```python
from build123d import *

# Parameters (mm, degrees)
F0_R     = 11
F1_DEPTH = 15


with BuildPart() as f1:
    # F0 (on Front) → F1 (new body)
    with BuildSketch(Plane.XZ):
        with BuildLine():
            Line((625, -53.625), (625, 53.625))
            Line((625, 53.625), (553.618176, 53.625))
            ThreePointArc((553.618176, 53.625), (525, 27.625), (496.381824, 53.625))
            Line((496.381824, 53.625), (478.618176, 53.625))
            ThreePointArc((478.618176, 53.625), (450, 27.625), (421.381824, 53.625))
            Line((421.381824, 53.625), (403.618176, 53.625))
            ThreePointArc((403.618176, 53.625), (375, 27.625), (346.381824, 53.625))
            Line((346.381824, 53.625), (328.618176, 53.625))
            ThreePointArc((328.618176, 53.625), (300, 27.625), (271.381824, 53.625))
            Line((271.381824, 53.625), (253.618176, 53.625))
            ThreePointArc((253.618176, 53.625), (225, 27.625), (196.381824, 53.625))
            Line((196.381824, 53.625), (178.618176, 53.625))
            ThreePointArc((178.618176, 53.625), (150, 27.625), (121.381824, 53.625))
            Line((121.381824, 53.625), (103.618176, 53.625))
            ThreePointArc((103.618176, 53.625), (75, 27.625), (46.381824, 53.625))
            Line((46.381824, 53.625), (28.618176, 53.625))
            ThreePointArc((28.618176, 53.625), (0, 27.625), (-28.618176, 53.625))
            Line((-28.618176, 53.625), (-46.381824, 53.625))
            ThreePointArc((-46.381824, 53.625), (-75, 27.625), (-103.618176, 53.625))
            Line((-103.618176, 53.625), (-121.381824, 53.625))
            ThreePointArc((-121.381824, 53.625), (-150, 27.625), (-178.618176, 53.625))
            Line((-178.618176, 53.625), (-196.381824, 53.625))
            ThreePointArc((-196.381824, 53.625), (-225, 27.625), (-253.618176, 53.625))
            Line((-253.618176, 53.625), (-271.381824, 53.625))
            ThreePointArc((-271.381824, 53.625), (-300, 27.625), (-328.618176, 53.625))
            Line((-328.618176, 53.625), (-346.381824, 53.625))
            ThreePointArc((-346.381824, 53.625), (-375, 27.625), (-403.618176, 53.625))
            Line((-403.618176, 53.625), (-421.381824, 53.625))
            ThreePointArc((-421.381824, 53.625), (-450, 27.625), (-478.618176, 53.625))
            Line((-478.618176, 53.625), (-496.381824, 53.625))
            ThreePointArc((-496.381824, 53.625), (-525, 27.625), (-553.618176, 53.625))
            Line((-553.618176, 53.625), (-625, 53.625))
            Line((-625, 53.625), (-625, -53.625))
            Line((-625, -53.625), (625, -53.625))
        make_face()
        with Locations((-350, -13.625)):
            Circle(F0_R, mode=Mode.SUBTRACT)
        with Locations((350, -13.625)):
            Circle(F0_R, mode=Mode.SUBTRACT)
        with Locations((-594.908628, 13.375)):
            Circle(F0_R, mode=Mode.SUBTRACT)
        with Locations((594.908628, 13.375)):
            Circle(F0_R, mode=Mode.SUBTRACT)
    extrude(amount=F1_DEPTH)


solid = f1.part
```
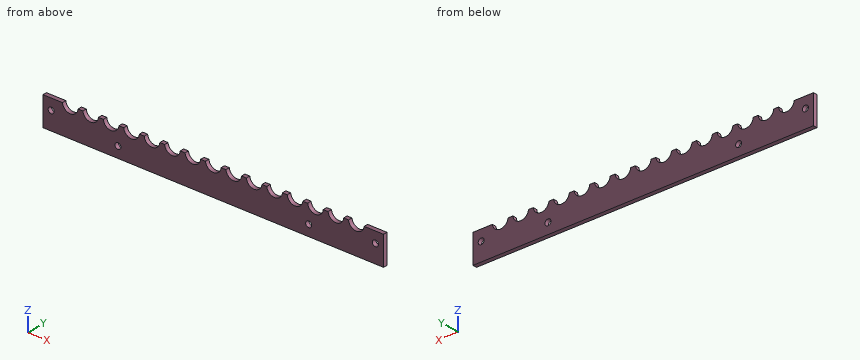
Verification items for the finished model (mm, model axes). Coordinates: 2 decimals unless noted, no trailing zeros. Order: outer loops, then holes, each group sorted by start corner. A loop starts at its lowest first (then second) coordinate and runs counter-clockwise, first axis right, second up. Notation, with made-up numbers: (4, 11.25) - (11, 11.25) arc R17 cw to (11, 26.25) - close; hole circle Ø9 at (-21, -35.5). An arc over 180 degrees is marked (long way). Return JSON: item names as keys, results as strings.
(1) Section check C-C, the plane x = 215. Record the cut outline in (y, z) (3 decimals).
Filled sheet:
{"outline": "(-15, -53.625) - (0, -53.625) - (0, 29.42) - (-15, 29.42) - close"}
(2) Section check A-A, the plane y = -10. Give the number of separate pieces and of enclosed holes in the cut face, and give its area (3 significant figures).
Filled sheet:
{"separate pieces": "1", "enclosed holes": "4", "area": "115,000 mm^2"}
(3) Go/stop test with flat-tipped pins: pin 1 (20 mm diameter, centred on x = -594.91, z = 13.38, fed in from -Y); pin 2 (8 mm diameter, centred on x = 14, y = -11.5, fed in from +Z). Record where each tip stops, or that it passes through.
Filled sheet:
{"pin 1": "passes through", "pin 2": "stops at z = 33.96"}
(4) Section check B-B, the plane x = -375.5. Record the cut outline in (y, z) (3 decimals), and give its area (3 significant figures).
Filled sheet:
{"outline": "(-15, -53.625) - (0, -53.625) - (0, 27.629) - (-15, 27.629) - close", "area": "1,220 mm^2"}
(5) Thickness scan on line 1 along X through (y, z) = (-0.25, -13); line 2 along X through (y, z) = (-13.75, -15.5); line 3 along Z through (x, y) = (-298, -10) (3 decimals). Record the ranges inside material, lowest first.
Filled sheet:
{"line 1": "x = -625 to -360.98, -339.02 to 339.02, 360.98 to 625", "line 2": "x = -625 to -360.84, -339.16 to 339.16, 360.84 to 625", "line 3": "z = -53.625 to 27.695"}
